For this review, take the finished solid that the model builds, in its own axes (mm). A direction names the side the tool comes from. Give positions to 0.01 mm unless a question says otherwise; leave off trailing zeros. Loops run counter-clockwise (first coordinate to the right, second up) from the corner with the lowest first, then second, coordinate; pieces in that order, holes last. Notation, with made-up numbers: (29, 36.5) -> (36, 36.5) arc R24 cw to (36, 63.5) -> close; hole circle Ø9 at (51, 58.5). An arc over 180 degrees is marked (long way). One line per question, with ' | ' between items. Start each with the question number.
(1) Wall thickness on probe 1 along X at (y, z) = (-0.2, 0); probe 2 along Z at (x, y) = (-88, -0.4); probe 3 along Z at (x, y) = (-109, 0): over which ranges is each line inside the solid? List them lowest first.
(2) Consider section A-A (x = -109). Write out the cut boundary in (y, z).
(3) Tool access review of faces 1 (the cylindrical face through (-36, 0, 0)), 2 (the cylindrical face through (-50.58, 0.01, 8.642)): name each direction out of +Z, -Z, +X, -X, +Y, -Y from which nothing blocks a thin tool from reaching the whole face with its end or side.
(4) Consider section C-C (y = -0.15). Give the number of separate pieces and of enclosed holes in the cut face, and give its area (3 significant figures).
(5) Draft analysis for pull direction Z (two halves, no side actions). For faces 3 (the flat face through (-66, -0.75, -4)), 4 (the cylindrical face through (-69.984, 0.01, -10.842)), 5 (the cylindrical face through (-43.647, -0.01, -1.736)), 6 (the cylindrical face through (-33, 0, 18.7)), state which applies: +Z half, -Z half, draft (parallel to the pull), parting line (faces both ways), or undercut.
(6) Consider section B-B (z = -19.75). Write out the cut boundary in (x, y).
(7) Consider section D-D (z = 16). Write out the cut boundary in (x, y).
(8) Insertion check: P1, Ø8, axis at x = -80.5, z = 17.5, coming from the -Y side; P2, Ø3.5, axis at x = -34.21, z = -19.75, coming from the +Y side. Each pin has a flat end and moves straight along its axis. Give the tip position at first contact, or say it passes through.
from build123d import *

# Parameters (mm, degrees)
SKETCH1_R                      = 3.5
BOSS_EXTRUDE1_DEPTH            = 0.75
F_3_2_3_2_DIAMETER_HOLE1_D     = 3.2
F_3_2_3_2_DIAMETER_HOLE1_DEPTH = 10
F_3_2_3_2_DIAMETER_HOLE1_TIP   = 0.96137699
CUT_EXTRUDE1_DEPTH             = 2.5
FILLET1_R                      = 2
SKETCH7_R                      = 9.5
CUT_EXTRUDE2_DEPTH             = 2.5000001


with BuildPart() as part:
    # Sketch1 → Boss-Extrude1 (new body, symmetric)
    with BuildSketch(Plane(origin=(0, 0, 0), x_dir=(1, 0, 0), z_dir=(0, 1, 0))):
        with BuildLine():
            ThreePointArc((-37.239092363, -21.5), (-43, 0), (-37.239092363, 21.5))
            ThreePointArc((-37.239092363, 21.5), (-36.658838331, 22.248681329), (-35.899079455, 22.81435343))
            ThreePointArc((-35.899079455, 22.81435343), (-70.492179883, 10.7556392), (-107.126701642, 10.839315166))
            ThreePointArc((-107.126701642, 10.839315166), (-120, 0), (-107.126701642, -10.839315166))
            ThreePointArc((-107.126701642, -10.839315166), (-70.492179883, -10.7556392), (-35.899079455, -22.81435343))
            ThreePointArc((-35.899079455, -22.81435343), (-36.658838331, -22.248681329), (-37.239092363, -21.5))
        make_face()
        with BuildLine():
            ThreePointArc((-31.176914536, 18), (-35.958003449, 16.718911087), (-37.239092363, 21.5))
            ThreePointArc((-37.239092363, 21.5), (-43, 0), (-37.239092363, -21.5))
            ThreePointArc((-37.239092363, -21.5), (-35.958003449, -16.718911087), (-31.176914536, -18))
            ThreePointArc((-31.176914536, -18), (-36, 0), (-31.176914536, 18))
        make_face()
        with Locations((-34.208003449, -19.75)):
            Circle(SKETCH1_R)
        with Locations((-34.208003449, 19.75)):
            Circle(SKETCH1_R)
    extrude(amount=BOSS_EXTRUDE1_DEPTH, both=True)

    # Ø3.2 (3.2) Diameter Hole1
    with Locations(Plane(origin=(0, 0.75, 0), x_dir=(1, 0, 0), z_dir=(0, 1, 0))):
        with Locations((-34.208003449, 19.75), (-34.208003449, -19.75), (-106.530652164, 14.288188173), (-106.530652164, -14.288188173)):
            Hole(F_3_2_3_2_DIAMETER_HOLE1_D / 2, depth=F_3_2_3_2_DIAMETER_HOLE1_DEPTH)
            with Locations((0, 0, -(F_3_2_3_2_DIAMETER_HOLE1_DEPTH + F_3_2_3_2_DIAMETER_HOLE1_TIP / 2))):  # 118° drill point
                Cone(0, F_3_2_3_2_DIAMETER_HOLE1_D / 2, F_3_2_3_2_DIAMETER_HOLE1_TIP, mode=Mode.SUBTRACT)

    # Sketch6 → Cut-Extrude1 (cut, through all)
    with BuildSketch(Plane(origin=(0, 0.75, 0), x_dir=(1, 0, 0), z_dir=(0, 1, 0))):
        with BuildLine():
            Line((-72.469338063, -3.369046694), (-49.802019621, 0))
            Line((-49.802019621, 0), (-72.469338063, 3.369046694))
            ThreePointArc((-72.469338063, 3.369046694), (-85.377857375, 2.290839769), (-98.326107181, 2.65857332))
            ThreePointArc((-98.326107181, 2.65857332), (-98, 0), (-98.326107181, -2.65857332))
            ThreePointArc((-98.326107181, -2.65857332), (-85.377857375, -2.290839769), (-72.469338063, -3.369046694))
        make_face()
        with BuildLine():
            Line((-66.096117167, 4.443764231), (-42.988154947, 1.009224591))
            ThreePointArc((-42.988154947, 1.009224591), (-42.467311238, 6.747405149), (-41.183985346, 12.36443897))
            ThreePointArc((-41.183985346, 12.36443897), (-53.416219701, 7.70010587), (-66.096117167, 4.443764231))
        make_face()
        with BuildLine():
            ThreePointArc((-41.183985346, -12.36443897), (-42.467311238, -6.747405149), (-42.988154947, -1.009224591))
            Line((-42.988154947, -1.009224591), (-66.096117167, -4.443764231))
            ThreePointArc((-66.096117167, -4.443764231), (-53.416219701, -7.70010587), (-41.183985346, -12.36443897))
        make_face()
    extrude(amount=-CUT_EXTRUDE1_DEPTH, mode=Mode.SUBTRACT)

    # Fillet1
    fillet1_edges = [part.edges().sort_by_distance(p)[0] for p in [
        (-98.326107181, 0, 2.65857332),
        (-98.326107181, 0, -2.65857332),
        (-72.469338063, 0, -3.369046694),
        (-49.802019621, 0, 0),
        (-72.469338063, 0, 3.369046694),
        (-41.183985346, 0, -12.36443897),
        (-42.988154947, 0, -1.009224591),
        (-66.096117167, 0, -4.443764231),
        (-42.988154947, 0, 1.009224591),
        (-41.183985346, 0, 12.36443897),
        (-66.096117167, 0, 4.443764231),
    ]]
    fillet(fillet1_edges, radius=FILLET1_R)

    # Sketch7 → Cut-Extrude2 (cut, through all)
    with BuildSketch(Plane(origin=(0, 0.75, 0), x_dir=(1, 0, 0), z_dir=(0, 1, 0))):
        with Locations((-109, 0)):
            Circle(SKETCH7_R)
    extrude(amount=-CUT_EXTRUDE2_DEPTH, mode=Mode.SUBTRACT)


solid = part.part
A:
1) probe 1: x = -120 to -118.5, -99.5 to -98, -61.41 to -36 | probe 2: z = -9.25 to -2.25, 2.25 to 9.25 | probe 3: z = -11 to -9.5, 9.5 to 11
2) outline: (-0.75, -11) -> (0.75, -11) -> (0.75, -9.5) -> (-0.75, -9.5) -> close; (-0.75, 9.5) -> (0.75, 9.5) -> (0.75, 11) -> (-0.75, 11) -> close
3) face 1: +X, +Y, -Y | face 2: +Y, -Y
4) separate pieces: 1 | enclosed holes: 6 | area: 1,450 mm^2
5) face 3: draft | face 4: -Z half | face 5: undercut | face 6: undercut
6) outline: (-41.88, -0.75) -> (-35.81, -0.75) -> (-35.81, 0.75) -> (-41.88, 0.75) -> close; (-32.61, -0.75) -> (-30.71, -0.75) -> (-30.71, 0.75) -> (-32.61, 0.75) -> close
7) outline: (-50.79, -0.75) -> (-32.25, -0.75) -> (-32.25, 0.75) -> (-50.79, 0.75) -> close
8) P1: passes through | P2: stops at y = 0.75
